```python
from build123d import *

# Parameters (mm, degrees)
BOSS_EXTRUDE1_DEPTH      = 7.8
BOSS_EXTRUDE1_DEPTH_BACK = 2.65
SKETCH1_W                = 299.45
SKETCH1_H                = 108.950000082
CUT_EXTRUDE1_START       = 2.65
SKETCH3_W                = 28.574999543
SKETCH3_H                = 19.050000082
SKETCH3_W_2              = 28.575000457
CUT_EXTRUDE1_DEPTH       = 3.15
CUT_EXTRUDE2_START       = -98.183332877
CUT_EXTRUDE2_OUTLINE_W   = 2.65
CUT_EXTRUDE2_OUTLINE_H   = 5.129290046
CUT_EXTRUDE2_DEPTH       = 5.2
CUT_EXTRUDE2_START_2     = 92.983332877
CUT_EXTRUDE2_2_OUTLINE_W = 2.65
CUT_EXTRUDE2_2_OUTLINE_H = 5.129290046
CUT_EXTRUDE2_2_DEPTH     = 5.2
CUT_EXTRUDE2_START_3     = -69.275
CUT_EXTRUDE2_3_OUTLINE_W = 2.65
CUT_EXTRUDE2_3_OUTLINE_H = 5.070709954
CUT_EXTRUDE2_3_DEPTH     = 5.2
CUT_EXTRUDE2_START_4     = 64.075
CUT_EXTRUDE2_4_OUTLINE_W = 2.65
CUT_EXTRUDE2_4_OUTLINE_H = 5.070709954
CUT_EXTRUDE2_4_DEPTH     = 5.2
FILLET1_R                = 5.25
FILLET2_R                = 1.55
FILLET3_R                = 0.25
CHAMFER1_SIZE            = 0.5
FILLET4_R                = 1
FILLET7_R                = 2.5


# Read off the part's stored shape, not the designer's step: Cut-Extrude2
with BuildPart() as part:
    # Sketch1 → Boss-Extrude1 (new, two sides: drawn at the far end of the back side and taken through both)
    with BuildSketch(Plane.XZ.offset(-BOSS_EXTRUDE1_DEPTH_BACK)):
        with Locations((0.005996207, -0.029290046)):
            Rectangle(SKETCH1_W, SKETCH1_H)
        Polygon((-143.369003793, 48.095709995), (143.380996207, 48.095709995), (143.380996207, -29.104290005), (114.80599575, -29.104290005), (114.80599575, -48.154290087), (-114.79400425, -48.154290087), (-114.79400425, -29.104290005), (-143.369003793, -29.104290005), align=None, mode=Mode.SUBTRACT)
    extrude(amount=BOSS_EXTRUDE1_DEPTH + BOSS_EXTRUDE1_DEPTH_BACK)

    # Sketch3 → Cut-Extrude1 (cut)
    with BuildSketch(Plane(origin=(0, 0, 0), x_dir=(1, 0, 0), z_dir=(0, 1, 0)).offset(CUT_EXTRUDE1_START)):
        with Locations((-129.081504021, 38.629290046)):
            Rectangle(SKETCH3_W, SKETCH3_H)
        with Locations((129.093495979, 38.629290046)):
            Rectangle(SKETCH3_W_2, SKETCH3_H)
    extrude(amount=-CUT_EXTRUDE1_DEPTH, mode=Mode.SUBTRACT)

    # Cut-Extrude2 outline → Cut-Extrude2 (cut)
    with BuildSketch(Plane.YZ.offset(CUT_EXTRUDE2_START)):
        with Locations((1.325, 50.660355018)):
            Rectangle(CUT_EXTRUDE2_OUTLINE_W, CUT_EXTRUDE2_OUTLINE_H)
    extrude(amount=CUT_EXTRUDE2_DEPTH, mode=Mode.SUBTRACT)

    # Cut-Extrude2 2 outline → Cut-Extrude2 2 (cut)
    with BuildSketch(Plane.YZ.offset(CUT_EXTRUDE2_START_2)):
        with Locations((1.325, 50.660355018)):
            Rectangle(CUT_EXTRUDE2_2_OUTLINE_W, CUT_EXTRUDE2_2_OUTLINE_H)
    extrude(amount=CUT_EXTRUDE2_2_DEPTH, mode=Mode.SUBTRACT)

    # Cut-Extrude2 3 outline → Cut-Extrude2 3 (cut)
    with BuildSketch(Plane.YZ.offset(CUT_EXTRUDE2_START_3)):
        with Locations((1.325, -50.689645064)):
            Rectangle(CUT_EXTRUDE2_3_OUTLINE_W, CUT_EXTRUDE2_3_OUTLINE_H)
    extrude(amount=CUT_EXTRUDE2_3_DEPTH, mode=Mode.SUBTRACT)

    # Cut-Extrude2 4 outline → Cut-Extrude2 4 (cut)
    with BuildSketch(Plane.YZ.offset(CUT_EXTRUDE2_START_4)):
        with Locations((1.325, -50.689645064)):
            Rectangle(CUT_EXTRUDE2_4_OUTLINE_W, CUT_EXTRUDE2_4_OUTLINE_H)
    extrude(amount=CUT_EXTRUDE2_4_DEPTH, mode=Mode.SUBTRACT)

    # Fillet1
    fillet1_edges = [part.edges().sort_by_distance(p)[0] for p in [
        (-149.719003793, -2.575, 54.445709995),
        (149.730996207, -2.575, 54.445709995),
        (149.730996207, -2.575, -54.504290087),
        (-149.719003793, -2.575, -54.504290087),
    ]]
    fillet(fillet1_edges, radius=FILLET1_R)

    # Fillet2
    fillet2_edges = [part.edges().sort_by_distance(p)[0] for p in [
        (-143.369003793, -2.575, 48.095709995),
        (143.380996207, -2.575, 48.095709995),
        (-143.369003793, -4.15, -29.104290005),
        (-114.79400425, -4.15, -48.154290087),
        (114.80599575, -4.15, -48.154290087),
        (143.380996207, -4.15, -29.104290005),
        (-143.369003793, 1.075, -48.154290087),
        (143.380996207, 1.075, -48.154290087),
    ]]
    fillet(fillet2_edges, radius=FILLET2_R)

    # Fillet3
    fillet3_edges = [part.edges().sort_by_distance(p)[0] for p in [
        (-149.719003793, 2.65, -0.029290046),
        (0.005996207, 2.65, -54.504290087),
        (0.005996207, 2.65, 54.445709995),
        (149.730996207, 2.65, -0.029290046),
        (-148.181314394, 2.65, 52.908020596),
        (148.193306808, 2.65, 52.908020596),
        (148.193306808, 2.65, -52.966600688),
        (-148.181314394, 2.65, -52.966600688),
    ]]
    fillet(fillet3_edges, radius=FILLET3_R)

    # Chamfer1
    chamfer1_edges = [part.edges().sort_by_distance(p)[0] for p in [
        (0.00599575, -7.8, -48.154290087),
        (143.380996207, -7.8, 9.495709995),
        (-143.369003793, -7.8, 9.495709995),
        (114.80599575, -7.8, -37.854290046),
        (0.005996207, -7.8, 48.095709995),
        (-128.306504021, -7.8, -29.104290005),
        (114.352011261, -7.8, -47.700305598),
        (142.927011718, -7.8, -28.650305516),
        (142.927011718, -7.8, 47.641725506),
        (-114.34001976, -7.8, -47.700305598),
        (-142.915019304, -7.8, -28.650305516),
        (-142.915019304, -7.8, 47.641725506),
        (-114.79400425, -7.8, -37.854290046),
        (128.318495979, -7.8, -29.104290005),
    ]]
    chamfer(chamfer1_edges, length=CHAMFER1_SIZE)

    # Fillet4
    fillet4_edges = [part.edges().sort_by_distance(p)[0] for p in [
        (-149.719003793, -7.8, -0.029290046),
        (0.005996207, -7.8, -54.504290087),
        (149.730996207, -7.8, -0.029290046),
        (0.005996207, -7.8, 54.445709995),
        (-148.181314394, -7.8, 52.908020596),
        (148.193306808, -7.8, 52.908020596),
        (148.193306808, -7.8, -52.966600688),
        (-148.181314394, -7.8, -52.966600688),
    ]]
    fillet(fillet4_edges, radius=FILLET4_R)

    # Fillet7
    fillet7_edges = [part.edges().sort_by_distance(p)[0] for p in [
        (-98.183332877, 1.325, 53.225000041),
        (-92.983332877, 1.325, 53.225000041),
        (92.983332877, 1.325, 53.225000041),
        (98.183332877, 1.325, 53.225000041),
        (69.275, 1.325, -53.225000041),
        (64.075, 1.325, -53.225000041),
        (-64.075, 1.325, -53.225000041),
        (-69.275, 1.325, -53.225000041),
        (-69.275, 1.325, -48.154290087),
        (-64.075, 1.325, -48.154290087),
        (69.275, 1.325, -48.154290087),
        (64.075, 1.325, -48.154290087),
        (92.983332877, 1.325, 48.095709995),
        (98.183332877, 1.325, 48.095709995),
        (-98.183332877, 1.325, 48.095709995),
        (-92.983332877, 1.325, 48.095709995),
    ]]
    fillet(fillet7_edges, radius=FILLET7_R)


solid = part.part
```
Input: part model. Units: mm. Frame: model coordinates. A direction names the side the tool comes from. Round coordinates to 2 decimals unless told otherwise and drop trailing zeros. Loops run counter-clockwise (first coordinate to the right, second up) from the corner with the lowest first, then second, coordinate; pieces in that order, holes last. Notation, with made-up numbers: (76.5, 10) -> (91.5, 10) arc R9 ccw to (91.5, 21) -> close; hole circle Ø4 at (83.25, 10.5). An arc over 180 degrees is marked (long way). One line per item, written item: value.
(1) Section A-A (x = 126.5). Return the cut outline in (y, z), plus the area to 3 significant figures.
Geometry check:
outline: (-7.8, -53.5) arc R1 ccw to (-6.8, -54.5) -> (2.4, -54.5) arc R0.25 ccw to (2.65, -54.25) -> (2.65, -48.15) -> (-0.5, -48.15) -> (-0.5, -29.1) -> (-7.3, -29.1) -> (-7.8, -29.6) -> close; (-7.8, 48.6) -> (-7.3, 48.1) -> (2.65, 48.1) -> (2.65, 54.2) arc R0.25 ccw to (2.4, 54.45) -> (-6.8, 54.45) arc R1 ccw to (-7.8, 53.45) -> close
area: 271 mm2
(2) Set-up query: faces 1 (the face through (-45, 2.65, 48.4)), 2 (the face through (129, -4, -29.104)), 3 (the face through (-96, 0, 50)). Return all of +Z, -Z, +X, -X, +Y, -Y with unobstructed straight access to the full face (end or side cutting, diameter ignored); none if empty.
Geometry check:
face 1: +Z, -Z, +X, -X, +Y
face 2: +Y, -Y
face 3: +Y
(3) Section D-D (x = 49). Return the cut outline in (y, z).
Geometry check:
outline: (-7.8, -53.5) arc R1 ccw to (-6.8, -54.5) -> (2.4, -54.5) arc R0.25 ccw to (2.65, -54.25) -> (2.65, -48.15) -> (-7.3, -48.15) -> (-7.8, -48.65) -> close; (-7.8, 48.6) -> (-7.3, 48.1) -> (2.65, 48.1) -> (2.65, 54.2) arc R0.25 ccw to (2.4, 54.45) -> (-6.8, 54.45) arc R1 ccw to (-7.8, 53.45) -> close
(4) Section B-B (z = 2.5). Return the cut outline in (x, y), plus the area to 3 significant figures.
Geometry check:
outline: (-149.72, -6.8) arc R1 ccw to (-148.72, -7.8) -> (-143.87, -7.8) -> (-143.37, -7.3) -> (-143.37, 2.65) -> (-149.47, 2.65) arc R0.25 ccw to (-149.72, 2.4) -> close; (143.38, -7.3) -> (143.88, -7.8) -> (148.73, -7.8) arc R1 ccw to (149.73, -6.8) -> (149.73, 2.4) arc R0.25 ccw to (149.48, 2.65) -> (143.38, 2.65) -> close
area: 132 mm2
(5) Material intervals for line 1 (Z direction, x = 34.5, y = -1); line 2 (Z direction, x = -126, y = -4.75); line 3 (X direction, y = -4, z = 25), sorted ascending. Write a range as [from, to].
Geometry check:
line 1: [-54.5, -48.15], [48.1, 54.45]
line 2: [-54.5, -29.1], [48.1, 54.45]
line 3: [-149.72, -143.37], [143.38, 149.73]
(6) Section C-C (y = -2.25). Return the cut outline in (x, z), plus the area to 3 significant figures.
Geometry check:
outline: (-149.72, -49.25) arc R5.25 ccw to (-144.47, -54.5) -> (144.48, -54.5) arc R5.25 ccw to (149.73, -49.25) -> (149.73, 49.2) arc R5.25 ccw to (144.48, 54.45) -> (-144.47, 54.45) arc R5.25 ccw to (-149.72, 49.2) -> close; hole (-143.37, -27.55) arc R1.55 ccw to (-141.82, -29.1) -> (-114.79, -29.1) -> (-114.79, -46.6) arc R1.55 ccw to (-113.24, -48.15) -> (113.26, -48.15) arc R1.55 ccw to (114.81, -46.6) -> (114.81, -29.1) -> (141.83, -29.1) arc R1.55 ccw to (143.38, -27.55) -> (143.38, 46.55) arc R1.55 ccw to (141.83, 48.1) -> (-141.82, 48.1) arc R1.55 ccw to (-143.37, 46.55) -> close
area: 6,090 mm2
(7) Pin query (flat end, axial travel): pin 1 (10.5 mm diameter, centred on x = 123.5, z = -42.5, fed in from +Y); pin 2 (5.5 mm diameter, centred on x = -67.5, z = -51, fed in from +Y). Return the tip coordinate at first contact, or that it passes through.
Geometry check:
pin 1: y = -0.5
pin 2: y = 2.65
(8) Mould query, pull axis X, two halves, no side actions, for faces 4 (the face through (-34, -7.8, -51)), 5 (the face through (-148.22, -2.26, -52.93)), 6 (the face through (128, -0.5, -40)). Classes: pulls with the +X half, pulls with the -X half, needs draft (parallel to the pull), parting line crosses it, or undercut.
Geometry check:
face 4: needs draft
face 5: pulls with the -X half
face 6: undercut
